```python
from build123d import *

# Parameters (mm, degrees)
IZIM1_R                     = 50
Y_KSEKLIK_EKSTR_ZYON1_DEPTH = 100
IZIM1_3_R                   = 57.5
IZIM1_3_R_2                 = 50
Y_KSEKLIK_EKSTR_ZYON2_DEPTH = 90
IZIM11_R                    = 31.5
Y_KSEKLIK_EKSTR_ZYON7_DEPTH = 120
IZIM12_W                    = 2.15
IZIM12_H                    = 5.230498787


with BuildPart() as part:
    # izim1 → Y_kseklik-Ekstr_zyon1 (new, symmetric)
    with BuildSketch(Plane(origin=(0, 0, 0), x_dir=(0, 0, -1), z_dir=(1, 0, 0))):
        Circle(IZIM1_R)
    extrude(amount=Y_KSEKLIK_EKSTR_ZYON1_DEPTH, both=True)

    # izim1_3 → Y_kseklik-Ekstr_zyon2 (add, symmetric)
    with BuildSketch(Plane(origin=(0, 0, 0), x_dir=(0, 0, -1), z_dir=(1, 0, 0))):
        with Locations(Location((0, 0, 0), (0, 0, 180))):
            Circle(IZIM1_3_R)
        Circle(IZIM1_3_R_2, mode=Mode.SUBTRACT)
    extrude(amount=Y_KSEKLIK_EKSTR_ZYON2_DEPTH, both=True)

    # izim11 → Y_kseklik-Ekstr_zyon7 (add)
    with BuildSketch(Plane(origin=(100, 0, 0), x_dir=(0, 0, -1), z_dir=(1, 0, 0))):
        with Locations(Location((0, 0, 0), (0, 0, 180))):
            Circle(IZIM11_R)
    y_kseklik_ekstr_zyon7 = extrude(amount=Y_KSEKLIK_EKSTR_ZYON7_DEPTH)

    # izim12 → Kes-D_nd_r1 (revolve, cut)
    with BuildSketch(Plane.XY, mode=Mode.PRIVATE) as kes_d_nd_r1_sk:
        with Locations((210.925, 32.615249394)):
            Rectangle(IZIM12_W, IZIM12_H)
    kes_d_nd_r1 = revolve(kes_d_nd_r1_sk.sketch.rotate(Axis((220, 0, 0), (-1, 0, 0)), 270), axis=Axis((220, 0, 0), (-1, 0, 0)), mode=Mode.SUBTRACT)

    # Aynalama6: Y_kseklik-Ekstr_zyon7, Kes-D_nd_r1 across plane
    add(y_kseklik_ekstr_zyon7.mirror(Plane(origin=(0, 0, 0), x_dir=(0, 0, 1), z_dir=(1, 0, 0))))
    add(kes_d_nd_r1.mirror(Plane(origin=(0, 0, 0), x_dir=(0, 0, 1), z_dir=(1, 0, 0))), mode=Mode.SUBTRACT)


solid = part.part
```
Geometry: final body of the model. Coordinates: model frame, mm. A direction names the side the tool comes from. Round coordinates to 2 decimals unless told otherwise and drop trailing zeros. Order: outer loops, then holes, each group sorted by start corner. A loop starts at its lowest first (then second) coordinate and runs counter-clockwise, first axis right, second up. Notation, with made-up numbers: (58.25, 78.5) -> (81.25, 78.5) arc R11 ccw to (81.25, 93.5) -> close; hole circle Ø10 at (38.5, -15). An arc over 180 degrees is marked (long way). Write each question's results on one line, items separated by ' | '.
Q1. Section query C-C (x = 32.5). Output: boundary loops of the cut face in (y, z), and give its area (3 significant figures).
Response values:
outline: circle Ø115 at (0, 0) | area: 10,400 mm²
Q2. Access query for faces 4 (the face through (211, -18, -24)), 5 (the face through (1.26, 56.133, -12.465)), 6 (the face through (220, 0, 0)), 7 (the face through (-215.944, -31.232, -4.101)), 8 (the face through (154.156, -31.232, -4.101)). Directions: +Z, -Z, +X, -X, +Y, -Y. A direction counts if a zero-diameter tool reaches every point of the face in a straight line with its end or side. Return the directions, or none.
Response values:
face 4: none | face 5: +X, -X | face 6: +Z, -Z, +X, +Y, -Y | face 7: -X | face 8: +X
Q3. Section query A-A (z = 44). Output: boundary loops of the cut face in (x, y), and give its area (3 significant figures).
Response values:
outline: (-100, -23.75) -> (-90, -23.75) -> (-90, -37.02) -> (90, -37.02) -> (90, -23.75) -> (100, -23.75) -> (100, 23.75) -> (90, 23.75) -> (90, 37.02) -> (-90, 37.02) -> (-90, 23.75) -> (-100, 23.75) -> close | area: 14,300 mm²
Q4. Pull-direction query (X, two-part tool) for faces 1 (the face through (95.07, 15.02, -47.69)), 2 (the face through (-90, -47.1, -17.3)), 3 (the face through (-209.85, -12, -28)); classes: released by +X, released by -X, zero draft, split by the parting line, or undercut.
Response values:
face 1: zero draft | face 2: released by -X | face 3: undercut
Q5. Pin query (flat end, axial travel): pin 1 Ø3 at (x, z) = (-99.5, 25.5) entering from -Y; pin 2 Ø6 at (x, z) = (-116.5, 23.5) entering from +Y; pin 3 Ø10 at (y, z) = (4.5, 38.5) entering from +X. Return the tip coordinate at first contact, or that it passes through.
Response values:
pin 1: y = -43.86 | pin 2: y = 23.92 | pin 3: x = 100
Q6. Section query B-B (x = -135). Output: boundary loops of the cut face in (y, z).
Response values:
outline: circle Ø63 at (0, 0)
Q7. Ray query, line 1 along X through (y, z) = (-28, -17.5); line 2 along Y through (x, z) = (-107.5, -0.5); line 3 along Y through (x, z) = (75, 1.5). Return the intervals inside material, ascending.
Response values:
line 1: -100 to 100 | line 2: -31.5 to 31.5 | line 3: -57.48 to 57.48
